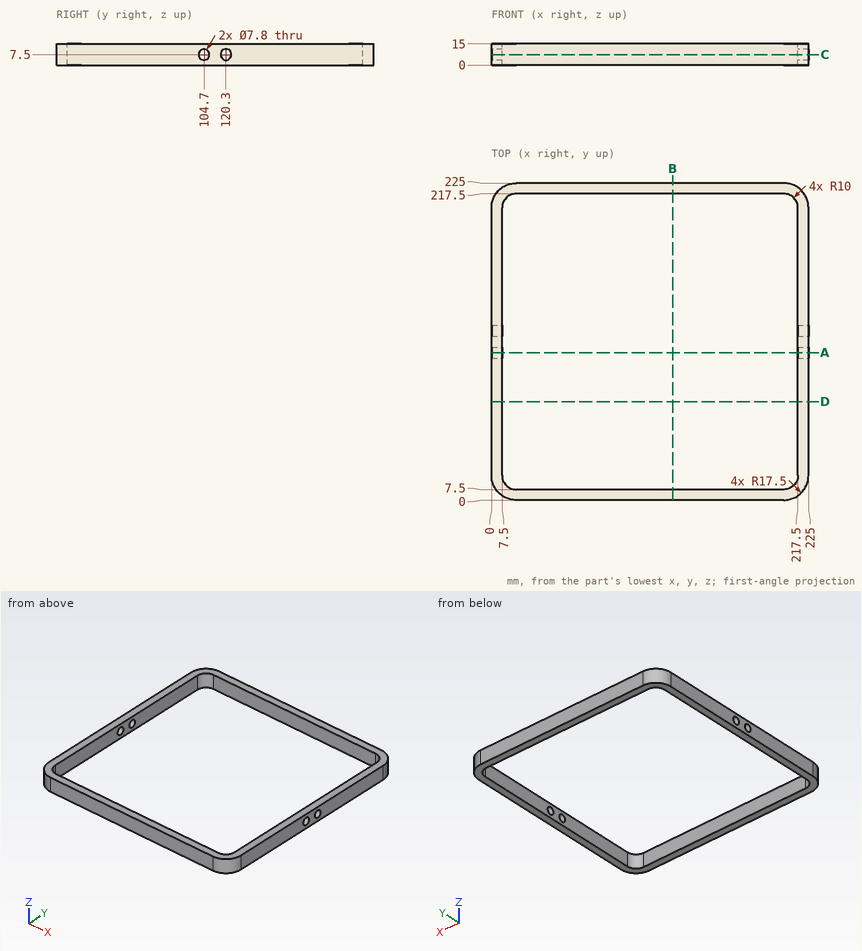
Answer from the drawing. Dimensions are ordinates in mm from the lowest x, y and z of the part. Give positions to 0.01 mm unless a question says otherwise; leave off trailing zeros. Write each loop counter-clockwise with the first axis right and the second up, starting at its lowest first coordinate (ties: lowest second). Pieces come first, ordered by that corner, then holes. Notation, with made-up numbers: (0.25, 24) -> (27.25, 24) arc R21 cw to (27.25, 28) -> close; hole circle Ø11 at (61.5, 41.5). An arc over 180 degrees is marked (long way). One line per question, with ' | ' between items. Start each with the question number.
1. Section C-C (z = 7.5) is taken. State how many separate pieces and enclosed holes the cut face has, plus the area to 3 significant figures.
2. Section A-A (y = 104.7) is taken. Determine the outline of the cut face in (x, z), plus the area to 3 significant figures.
3. Given pin 1 Ø3 at (y, z) = (174, 5.5) entering from -X, flat-ended and moving along its own axis, determine where the tip first touches the part or whether it passes through.
4. Section B-B (x = 128.5) is taken. Determine the outline of the cut face in (y, z).
5. Find the intervals of material crossed by probe 1 along X at (y, z) = (131.5, 10.25); probe 2 along Z at (x, y) = (220, 120), in increasing order.
Response values:
1) separate pieces: 4 | enclosed holes: 0 | area: 6,110 mm2
2) outline: (0, 0) -> (7.5, 0) -> (7.5, 3.6) -> (0, 3.6) -> close; (0, 11.4) -> (7.5, 11.4) -> (7.5, 15) -> (0, 15) -> close; (217.5, 0) -> (225, 0) -> (225, 3.6) -> (217.5, 3.6) -> close; (217.5, 11.4) -> (225, 11.4) -> (225, 15) -> (217.5, 15) -> close | area: 108 mm2
3) pin 1: x = 0
4) outline: (0, 0) -> (7.5, 0) -> (7.5, 15) -> (0, 15) -> close; (217.5, 0) -> (225, 0) -> (225, 15) -> (217.5, 15) -> close
5) probe 1: 0 to 7.5, 217.5 to 225 | probe 2: 0 to 3.61, 11.39 to 15
